The model under review builds one solid part; all positions refer to its coordinate system, in mm. Face numbers are marked on the shaded views. A direction names the side the tool comes from. Round coordinates to 2 decimals unless told otherwise and drop trailing zeros. Write each loop counter-clockwise with the first axis right and the second up, starting at its lowest first coordinate (ties: lowest second). Pieces come first, ordered by that corner, then holes.
Item 1: Add section A-A (y = 8). Give the boundary of the cut face in (x, z).
Item 2: Draft analysis for pull direction X (two halves, no side actions). For the marked faces 3 and 4, state which applies: +X half, -X half, draft (parallel to the pull), parting line (faces both ways), or undercut.
Item 3: Add section C-C (z = 15). Give the boundary of the cut face in (x, y), plus the area to 3 significant figures.
Item 4: Add section B-B (x = 35.5). Give the boundary of the cut face in (y, z).
Item 5: Machinability: for the marked faces 1 and 2, which of the approach directions +Z, -Z, +X, -X, +Y, -Y give a long, thin tool a straight path to every point of the face, cutting with its end or side? Answer none if there is none.
Item 6: Clearance check with flat-ended pins moving along their axes: pin 1 Ø1.6 at (x, y) = (-41.5, 36) entering from -Z; pin 2 Ø6 at (x, z) = (-16, -24) entering from +Y; pin 3 Ø9 at (y, z) = (9.5, -6.5) entering from +X. State where each tip first meets the part, or that it passes through.
Item 7: To check wall thickness, follow L1, parallel to Z at x = 17.5, y = 18.5; L2, parallel to Y at x = -40.95, z = 42.5; L3, parallel to X at y = 28.5, z = 36.5. State the ranges of each line that lie inside material, in increasing order.
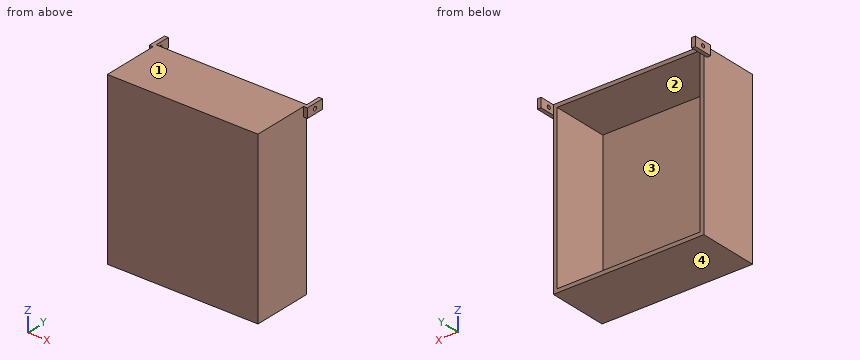
```python
from build123d import *

# Parameters (mm, degrees)
SKETCH1_W           = 80
SKETCH1_H           = 90
BOSS_EXTRUDE1_DEPTH = 2
SKETCH2_W           = 80
SKETCH2_H           = 90
SKETCH2_W_2         = 76
SKETCH2_H_2         = 86
BOSS_EXTRUDE2_DEPTH = 30
SKETCH4_W           = 5
SKETCH4_H           = 10
SKETCH4_R           = 1
BOSS_EXTRUDE3_DEPTH = 2
BOSS_EXTRUDE4_START = 2
SKETCH5_W           = 5
SKETCH5_H           = 10
SKETCH5_R           = 1
BOSS_EXTRUDE4_DEPTH = 2


with BuildPart() as part:
    # Sketch1 → Boss-Extrude1 (new body)
    with BuildSketch(Plane(origin=(0, 0, 0), x_dir=(1, 0, 0), z_dir=(0, 1, 0))):
        Rectangle(SKETCH1_W, SKETCH1_H)
    extrude(amount=BOSS_EXTRUDE1_DEPTH)

    # Sketch2 → Boss-Extrude2 (add)
    with BuildSketch(Plane(origin=(0, 2, 0), x_dir=(1, 0, 0), z_dir=(0, 1, 0))):
        Rectangle(SKETCH2_W, SKETCH2_H)
        Rectangle(SKETCH2_W_2, SKETCH2_H_2, mode=Mode.SUBTRACT)
    extrude(amount=BOSS_EXTRUDE2_DEPTH)

    # Sketch4 → Boss-Extrude3 (add)
    with BuildSketch(Plane(origin=(40, 0, 0), x_dir=(0, 0, -1), z_dir=(1, 0, 0))):
        with Locations((-42.5, 35)):
            Rectangle(SKETCH4_W, SKETCH4_H)
        with Locations((-42.5, 35)):
            Circle(SKETCH4_R, mode=Mode.SUBTRACT)
    extrude(amount=BOSS_EXTRUDE3_DEPTH)

    # Sketch5 → Boss-Extrude4 (add)
    with BuildSketch(Plane.ZY.offset(40).offset(BOSS_EXTRUDE4_START)):
        with Locations((42.5, 35)):
            Rectangle(SKETCH5_W, SKETCH5_H)
        with Locations(Location((42.5, 35, 0), (0, 0, 180))):
            Circle(SKETCH5_R, mode=Mode.SUBTRACT)
    extrude(amount=-BOSS_EXTRUDE4_DEPTH)


solid = part.part
```
Numbers:
1. outline: (-40, -45) - (40, -45) - (40, 45) - (-40, 45) - close; hole (-38, -43) - (38, -43) - (38, 43) - (-38, 43) - close
2. face 3: undercut
2. face 4: draft
3. outline: (-40, 0) - (40, 0) - (40, 32) - (38, 32) - (38, 2) - (-38, 2) - (-38, 32) - (-40, 32) - close
3. area: 280 mm2
4. outline: (0, -45) - (32, -45) - (32, -43) - (2, -43) - (2, 43) - (32, 43) - (32, 45) - (0, 45) - close
5. face 1: +Z, +X, -X, +Y, -Y
5. face 2: +Y
6. pin 1: stops at z = 40
6. pin 2: stops at y = 2
6. pin 3: stops at x = 40
7. L1: z = -45 to -43, 43 to 45
7. L2: y = 30 to 34, 36 to 40
7. L3: x = -40 to -38, 38 to 40
